Input: dimensioned drawing with shaded views. Units: mm. Origin: part minimum x, y, z. Coordinates: 2 decimals unless noted, no trailing zeros. Order: outer loops, then holes, each group sorted by start corner. A loop starts at its lowest first (then second) coordinate and runs counter-clockwise, first axis right, second up. Notation, with made-up numbers: M -19.5,48 L 2.5,48 A12 ccw 2.5,70 Z; hole C 84.5,-27 d11. An arc over 180 degrees is marked long. Write item = value, one per line.
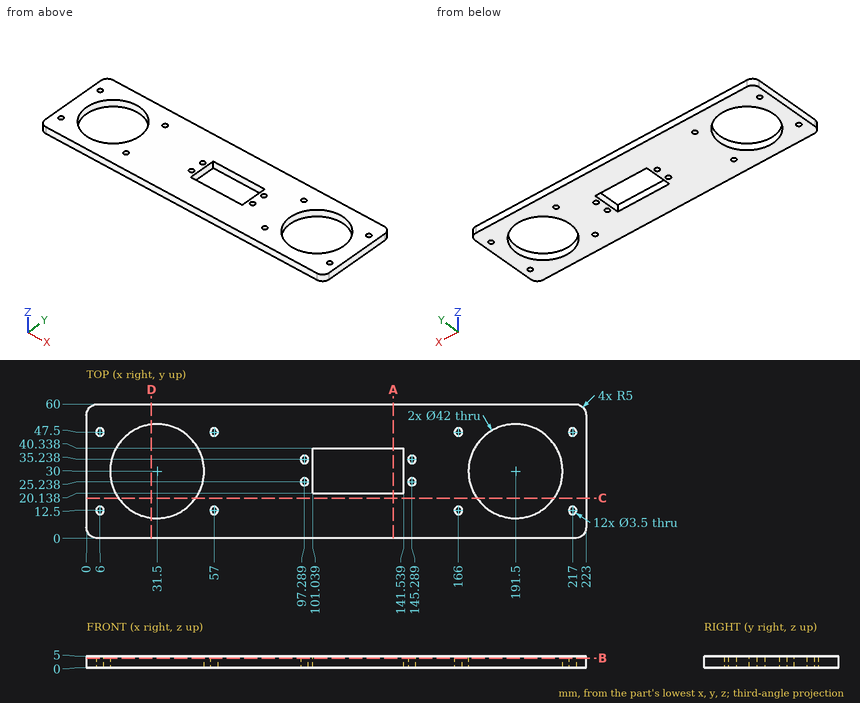
1) Section A-A, the plane x = 137. Return loops of the section in (y, z), and give its area (3 significant figures).
Numbers:
outline = M 0,0 L 20.14,0 L 20.14,5 L 0,5 Z; M 40.34,0 L 60,0 L 60,5 L 40.34,5 Z
area = 199 mm²
2) Section B-B, the plane z = 4.2. Give the number of separate pieces and of enclosed holes in the cut face, and give its area (3 significant figures).
Numbers:
separate_pieces = 1
enclosed_holes = 15
area = 9,650 mm²
3) Line query: L1, parallel to Y at x = 217, z = 1.7; L2, parallel to Y at x = 97, z = 2.15; L3, parallel to X at y = 41, z = 1.1. Output: solid intervals per line, ascending.
Numbers:
L1 = 0 to 10.75, 14.25 to 45.75, 49.25 to 60
L2 = 0 to 23.51, 26.96 to 33.51, 36.96 to 60
L3 = 0 to 13.61, 49.39 to 173.61, 209.39 to 223
4) Section C-C, the plane y = 18. Return loops of the section in (x, z).
Numbers:
outline = M 0,0 L 14.27,0 L 14.27,5 L 0,5 Z; M 48.73,0 L 174.27,0 L 174.27,5 L 48.73,5 Z; M 208.73,0 L 223,0 L 223,5 L 208.73,5 Z
5) Section D-D, the plane x = 29. Return loops of the section in (y, z), and give its area (3 significant figures).
Numbers:
outline = M 0,0 L 9.15,0 L 9.15,5 L 0,5 Z; M 50.85,0 L 60,0 L 60,5 L 50.85,5 Z
area = 91.5 mm²
